Model file for the job. Use its own axes, mm. A direction names the side the tool comes from. Coordinates: 2 decimals unless noted, no trailing zeros. Order: outer loops, then holes, each group sorted by start corner. A loop starts at its lowest first (then second) coordinate and runs counter-clockwise, first axis right, second up. Notation, with made-up numbers: (44, 22) -> (103, 22) arc R30 ccw to (103, 45) -> close; hole circle Ø7 at (79, -30). An arc over 180 degrees is marked (long way). Use CSV: the item, a comma, the result in double quotes. Start each with the question number.
(1) Tool access for faces 1 (the cylindrical face through (21.455, 19.645, 9.86)), 2 (the flat face through (24.707, 25.206, 10.14)), 3 (the flat face through (25, 16.546, 10)): list every direction of +Z, -Z, +X, -X, +Y, -Y with a clear straight run to the whole face (end or side of a thin tool).
(2) Probe L1, parallel to X at y = 2.3, z = -4; L2, parallel to X at y = 22, z = 2.5; L3, parallel to Y at x = 30.75, z = 5.75. List the from-to ranges inside material, lowest first.
(3) Pin check, flat tips, straight feed: pin 1 Ø1.5 at (x, z) = (16, 1.5) entering from +Y; pin 2 Ø4 at (x, y) = (34.5, 12) entering from -Z; pin 3 Ø4 at (x, y) = (25, 20) entering from +Z; pin 4 Ø3.5 at (y, z) = (20.5, 7) entering from -X. Stop position of each tip, or through.
(4) Cut at A-A on x = 16.5. Write the cut outline in (y, z), plus the area to 3 significant figures.
(5) Cut at B-B on z = -4. Write the cut outline in (x, y).
(6) Pull direction X, two halves, no side cores. Call faces 4 (the flat face through (20.225, 28.108, 10.14)), 5 (the cylindrical face through (22.53, 29.3, 10.14)), 6 (the flat face through (21, 16, 0)), 7 (the cylindrical face through (32.377, 1.521, -4.249)): pulls with the +X half, pulls with the -X half, needs draft (parallel to the pull), parting line crosses it, or undercut.
```python
from build123d import *

# Parameters (mm, degrees)
SCHIZZO1_W                     = 50
SCHIZZO1_H                     = 3
ESTRUSIONE_ESTRUSIONE1_DEPTH   = 20
ESTRUSIONE_ESTRUSIONE2_DEPTH   = 20
ESTRUSIONE_ESTRUSIONE2_2_DEPTH = 20
RACCORDO2_R                    = 6
RACCORDO3_DEPTH                = 20
RACCORDO4_R                    = 6
RACCORDO5_R                    = 6
RACCORDO7_R                    = 2
RACCORDO8_R                    = 2
SCHIZZO5_W                     = 11.5
SCHIZZO5_H                     = 20
TAGLIO_ESTRUSIONE2_DEPTH       = 3
ESTRUSIONE_ESTRUSIONE7_DEPTH   = 20
SCHIZZO12_W                    = 27
SCHIZZO12_H                    = 7
SCHIZZO12_R                    = 1.15
ESTRUSIONE_ESTRUSIONE9_DEPTH   = 3


with BuildPart() as part:
    # Schizzo1 → Estrusione-Estrusione1 (new body)
    with BuildSketch(Plane.XY):
        with Locations((25, 1.5)):
            Rectangle(SCHIZZO1_W, SCHIZZO1_H)
    extrude(amount=ESTRUSIONE_ESTRUSIONE1_DEPTH)

    # Schizzo5 → Taglio-Estrusione2 (cut)
    with BuildSketch(Plane(origin=(0, 3, 0), x_dir=(1, 0, 0), z_dir=(0, 1, 0))):
        with Locations((5.75, -10)):
            Rectangle(SCHIZZO5_W, SCHIZZO5_H)
        with Locations((44.25, -10)):
            Rectangle(SCHIZZO5_W, SCHIZZO5_H)
    extrude(amount=-TAGLIO_ESTRUSIONE2_DEPTH, mode=Mode.SUBTRACT)



with BuildPart() as body_2:
    # Schizzo2 → Estrusione-Estrusione2 (new body)
    with BuildSketch(Plane.XY.offset(20)):
        Polygon((12, 3), (21.667680152, 19.610006491), (21.667680152, 25.610006491), (18.742038116, 30.677367142), (23.742038116, 30.677367142), (24.8, 24.677367142), (23.500961894, 23.927367142), (24.8, 22.837344747), (24.8, 19.837344747), (15, 3), align=None)
    extrude(amount=-ESTRUSIONE_ESTRUSIONE2_DEPTH)

    # Raccordo2
    # the kernel refuses this fillet: 6 mm, written as the material it takes off along each edge
    with BuildSketch(Plane(origin=(23.742038116, 30.677367142, 32.586494468), x_dir=(-1, 0, 0), z_dir=(0, 0, -1))) as raccordo2_piece_1:
        with BuildLine():
            CenterArc((RACCORDO2_R * 0.839099631177, -RACCORDO2_R), RACCORDO2_R, 90, 80)
            Line((-RACCORDO2_R * 0.145708121835, -RACCORDO2_R * 0.826351822333), (0, 0))
            Line((0, 0), (RACCORDO2_R * 0.839099631177, 0))
        make_face()
    extrude(amount=45.172988935, mode=Mode.SUBTRACT)

    # Raccordo5
    raccordo5_edges = [body_2.edges().sort_by_distance(p)[0] for p in [
        (21.667680152, 19.610006491, 10),
    ]]
    fillet(raccordo5_edges, radius=RACCORDO5_R)

    # Raccordo8
    raccordo8_edges = [body_2.edges().sort_by_distance(p)[0] for p in [
        (15, 3, 10),
    ]]
    fillet(raccordo8_edges, radius=RACCORDO8_R)

    # Schizzo9 → Estrusione-Estrusione7 (add)
    with BuildSketch(Plane.XY.offset(20)):
        Polygon((24.564100135, 19.432046037), (22.884294771, 16.545978484), (26.884294771, 16.545978484), (25.204489408, 19.432046037), align=None)
    extrude(amount=-ESTRUSIONE_ESTRUSIONE7_DEPTH)


with BuildPart() as body_3:
    # Schizzo2 → Estrusione-Estrusione2 2 (new body)
    with BuildSketch(Plane.XY.offset(20)):
        Polygon((26.499038106, 23.927367142), (25.2, 22.837344747), (25.2, 19.837344747), (35, 3), (38, 3), (28.332319848, 19.610006491), (28.332319848, 25.610006491), (31.257961884, 30.677367142), (26.257961884, 30.677367142), (25.2, 24.677367142), align=None)
    extrude(amount=-ESTRUSIONE_ESTRUSIONE2_2_DEPTH)

    # Raccordo3: read off the stored shape, not the designer's step
    # Raccordo3 outline → Raccordo3 (cut)
    with BuildSketch(Plane.XY):
        with BuildLine():
            add(Edge.make_bspline(
                [(31.257961884, 30.677367142), (26.252870263, 30.648491125), (25.38373076, 25.719356061)],
                knots=[0, 0, 0, 1, 1, 1], degree=2, weights=[1, 0.767895459, 1]))
            Line((31.257961884, 30.677367142), (26.257961884, 30.677367142))
            Line((26.257961884, 30.677367142), (25.38373076, 25.719356061))
        make_face()
    extrude(amount=RACCORDO3_DEPTH, mode=Mode.SUBTRACT)

    # Raccordo4
    raccordo4_edges = [body_3.edges().sort_by_distance(p)[0] for p in [
        (28.332319848, 19.610006491, 10),
    ]]
    fillet(raccordo4_edges, radius=RACCORDO4_R)

    # Raccordo7
    raccordo7_edges = [body_3.edges().sort_by_distance(p)[0] for p in [
        (35, 3, 10),
    ]]
    fillet(raccordo7_edges, radius=RACCORDO7_R)


with BuildPart() as part_1:
    add(part.part)

    add(body_2.part)  # Estrusione-Estrusione9 merges body 2

    add(body_3.part)  # Estrusione-Estrusione9 merges body 3
    # Schizzo12 → Estrusione-Estrusione9 (add)
    with BuildSketch(Plane(origin=(0, 3, 0), x_dir=(1, 0, 0), z_dir=(0, 1, 0))):
        with Locations((25, 3.5)):
            Rectangle(SCHIZZO12_W, SCHIZZO12_H)
        with Locations(Location((16.5, 4, 0), (0, 0, 270))):
            Circle(SCHIZZO12_R, mode=Mode.SUBTRACT)
        with Locations(Location((33.5, 4, 0), (0, 0, 270))):
            Circle(SCHIZZO12_R, mode=Mode.SUBTRACT)
    extrude(amount=-ESTRUSIONE_ESTRUSIONE9_DEPTH)


solid = part_1.part
```
Outcome:
1,face 1,"+Z, -Z, -X"
1,face 2,"+Z, -Z, +Y"
1,face 3,"+Z, -Z"
2,L1,"11.5 to 15.35, 17.65 to 32.35, 34.65 to 38.5"
2,L2,"21.67 to 24.8, 25.2 to 28.33"
2,L3,"0 to 3, 10.3 to 15.46, 29.8 to 30.65"
3,pin 1,"y = 11.16"
3,pin 2,"z = 0"
3,pin 3,"z = 20"
3,pin 4,"x = 21.13"
4,outline,"(0, -7) -> (3, -7) -> (3, -5.15) -> (0, -5.15) -> close; (0, -2.85) -> (3, -2.85) -> (3, 20) -> (0, 20) -> close; (5.58, 0) -> (10.73, 0) -> (10.73, 20) -> (5.58, 20) -> close"
4,area,"177 mm2"
5,outline,"(11.5, 0) -> (15.35, 0) -> (15.35, 3) -> (11.5, 3) -> close; (17.65, 0) -> (32.35, 0) -> (32.35, 3) -> (17.65, 3) -> close; (34.65, 0) -> (38.5, 0) -> (38.5, 3) -> (34.65, 3) -> close"
6,face 4,"pulls with the -X half"
6,face 5,"undercut"
6,face 6,"needs draft"
6,face 7,"undercut"
